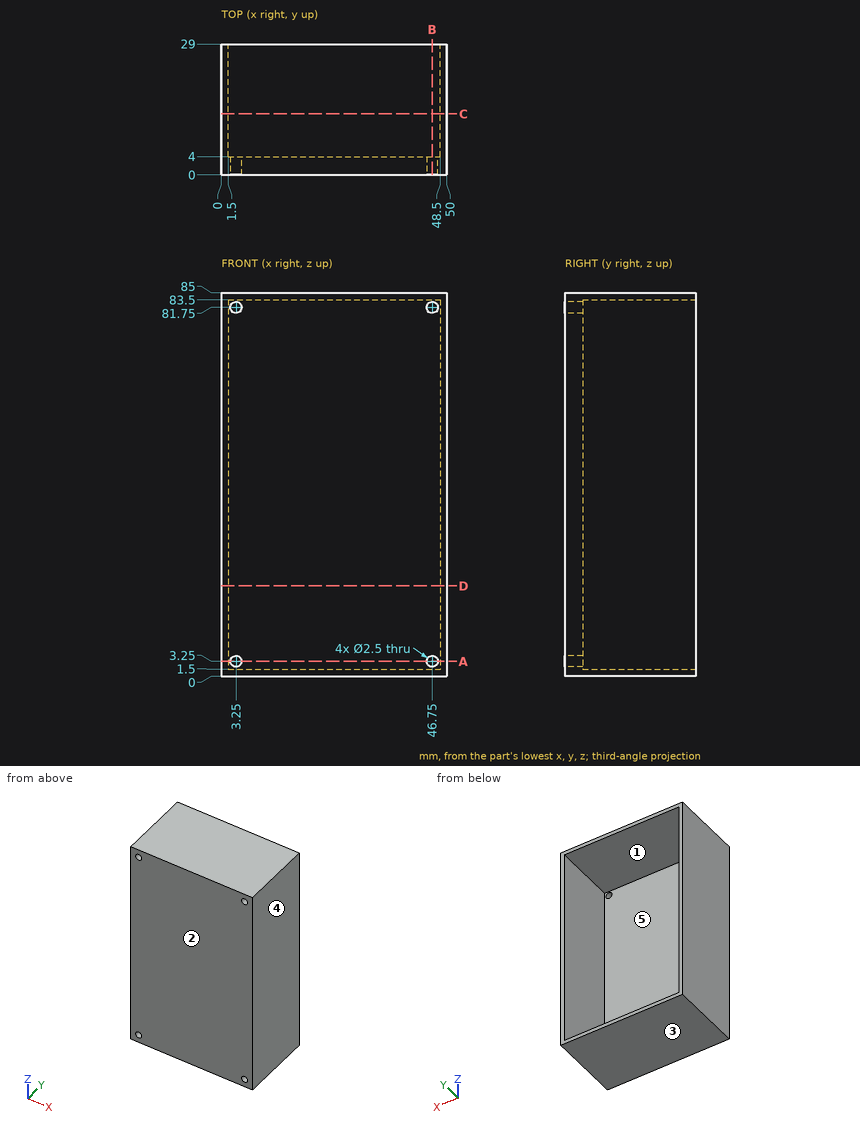
Answer from the drawing. Dimensions are ordinates in mm from the lowest x, y and z of the part. A direction names the side the tool comes from. Coordinates: 2 decimals unless noted, no trailing zeros. Order: outer loops, then holes, each group sorted by start corner. A loop starts at its lowest first (then second) coordinate and runs counter-clockwise, first axis right, second up. Notation, with made-up numbers: M 77,75 L 115,75 A12 ccw 115,86 Z; hole C 18,32.5 d11. An arc over 180 degrees is marked long. Put each result on its own line as item: value. Start each with the question number.
Item 1: For the marked faces 1 and 2, determine the directions among +Z, -Z, +X, -X, +Y, -Y from which every point of the face is accessible in a straight line to the end or side of a thin tool.
Item 2: Section C-C, the plane y = 13.5 is taken. Determine the outline of the cut face in (x, z).
Item 3: Section A-A, the plane z = 3.25 is taken. Determine the outline of the cut face in (x, y), plus the area to 3 significant figures.
Item 4: Section D-D, the plane z = 20 is taken. Determine the outline of the cut face in (x, y), plus the area to 3 significant figures.
Item 5: Given pin 1 Ø3 at (x, z) = (29, 35) entering from +Y; pin 2 Ø2 at (x, z) = (3.25, 81.75) entering from +Y, each flat-ended and moving along its own axis, determine where each tip first touches the part or whether it passes through.
Item 6: Consider probe 1 along X at (y, z) = (1.8, 3.25); probe 2 along Z at (x, y) = (46.75, 1.7); probe 3 along Z at (x, y) = (36, 19). Determine where each line is inside the solid, lowest interval first. Write a range as [from, to].
Item 7: Section B-B, the plane x = 46.75 is taken. Determine the outline of the cut face in (y, z).
Item 8: The mould has two halves that part along X. Classify the marked faces 3, 4 and 5: +X half, -X half, draft (parallel to the pull), parting line (faces both ways), or undercut.
Computed:
1. face 1: +Y
1. face 2: +Z, -Z, +X, -X, -Y
2. outline: M 0,0 L 50,0 L 50,85 L 0,85 Z; hole M 1.5,1.5 L 48.5,1.5 L 48.5,83.5 L 1.5,83.5 Z
3. outline: M 0,0 L 2,0 L 2,4 L 1.5,4 L 1.5,29 L 0,29 Z; M 4.5,0 L 45.5,0 L 45.5,4 L 4.5,4 Z; M 48,0 L 50,0 L 50,29 L 48.5,29 L 48.5,4 L 48,4 Z
3. area: 255 mm2
4. outline: M 0,0 L 50,0 L 50,29 L 48.5,29 L 48.5,4 L 1.5,4 L 1.5,29 L 0,29 Z
4. area: 275 mm2
5. pin 1: stops at y = 4
5. pin 2: passes through
6. probe 1: x = [0, 2], [4.5, 45.5], [48, 50]
6. probe 2: z = [0, 2], [4.5, 80.5], [83, 85]
6. probe 3: z = [0, 1.5], [83.5, 85]
7. outline: M 0,0 L 29,0 L 29,1.5 L 4,1.5 L 4,2 L 0,2 Z; M 0,4.5 L 4,4.5 L 4,80.5 L 0,80.5 Z; M 0,83 L 4,83 L 4,83.5 L 29,83.5 L 29,85 L 0,85 Z
8. face 3: draft
8. face 4: +X half
8. face 5: undercut
